from build123d import *

# Parameters (mm, degrees)
SKETCH1_R           = 9.525
BOSS_EXTRUDE1_DEPTH = 7.62
SKETCH2_R           = 3.175
CUT_EXTRUDE1_DEPTH  = 16.476293161
CUT_SWEEP5_PITCH    = 4.98602


with BuildPart() as part:
    # Sketch1 → Boss-Extrude1 (new body)
    with BuildSketch(Plane.XY):
        with Locations(Location((0, 0, 0), (0, 0, 180))):
            Circle(SKETCH1_R)
    extrude(amount=BOSS_EXTRUDE1_DEPTH)

    # Sketch2 → Cut-Extrude1 (cut, through all)
    with BuildSketch(Plane.XY.offset(7.62)):
        Circle(SKETCH2_R)
    extrude(amount=-CUT_EXTRUDE1_DEPTH, mode=Mode.SUBTRACT)

    # Cut-Sweep5: arcs per turn and ends read off the stored shape
    # Cut-Sweep5: the profile of Sketch6 screwed along a left-hand helix through 2.5 turns, 12 arcs to a turn; built about Z, then put on its axis
    cut_sweep5_z = Axis((0, 0, 0), (0, 0, 1))
    cut_sweep5_corners = [(10.033, 2e-08, -1.522198128), (10.033, 2e-08, 1.525801872), (8.509, 1.7e-08, 0.255801872), (8.509, 1.7e-08, -0.252198128)]
    with BuildLine(mode=Mode.PRIVATE) as cut_sweep5_profile:
        Line(cut_sweep5_corners[0], cut_sweep5_corners[1])
        Line(cut_sweep5_corners[1], cut_sweep5_corners[2])
        Line(cut_sweep5_corners[2], cut_sweep5_corners[3])
        Line(cut_sweep5_corners[3], cut_sweep5_corners[0])
    cut_sweep5_cap = Face(cut_sweep5_profile.wire())
    cut_sweep5_turn_angles = [0, -15, -30, -45, -60, -75, -90, -105, -120, -135, -150, -165, -180, -195, -210, -225, -240, -255, -270, -285, -300, -315, -330, -345, -360]
    cut_sweep5_turn_weights = [1, 0.9659258262890683, 1, 0.9659258262890683, 1, 0.9659258262890683, 1, 0.9659258262890683, 1, 0.9659258262890683, 1, 0.9659258262890683, 1, 0.9659258262890683, 1, 0.9659258262890683, 1, 0.9659258262890683, 1, 0.9659258262890683, 1, 0.9659258262890683, 1, 0.9659258262890683, 1]
    cut_sweep5_turn_rails = [Edge.make_bspline([Vector(p[0], p[1], 0).rotate(cut_sweep5_z, cut_sweep5_turn_angles[k]) / cut_sweep5_turn_weights[k] + Vector(0, 0, p[2] + -CUT_SWEEP5_PITCH * cut_sweep5_turn_angles[k] / 360) for k in range(25)], [0, 0, 0, 1, 1, 2, 2, 3, 3, 4, 4, 5, 5, 6, 6, 7, 7, 8, 8, 9, 9, 10, 10, 11, 11, 12, 12, 12], 2, cut_sweep5_turn_weights) for p in cut_sweep5_corners]
    cut_sweep5_turn_sides = [Face.make_surface_from_curves(cut_sweep5_turn_rails[p[0]], cut_sweep5_turn_rails[p[1]]) for p in [(0, 1), (1, 2), (2, 3), (3, 0)]]
    cut_sweep5_last_angles = [-720, -735, -750, -765, -780, -795, -810, -825, -840, -855, -870, -885, -900]
    cut_sweep5_last_weights = [1, 0.9659258262890683, 1, 0.9659258262890683, 1, 0.9659258262890683, 1, 0.9659258262890683, 1, 0.9659258262890683, 1, 0.9659258262890683, 1]
    cut_sweep5_last_rails = [Edge.make_bspline([Vector(p[0], p[1], 0).rotate(cut_sweep5_z, cut_sweep5_last_angles[k]) / cut_sweep5_last_weights[k] + Vector(0, 0, p[2] + -CUT_SWEEP5_PITCH * cut_sweep5_last_angles[k] / 360) for k in range(13)], [0, 0, 0, 1, 1, 2, 2, 3, 3, 4, 4, 5, 5, 6, 6, 6], 2, cut_sweep5_last_weights) for p in cut_sweep5_corners]
    cut_sweep5_last_sides = [Face.make_surface_from_curves(cut_sweep5_last_rails[p[0]], cut_sweep5_last_rails[p[1]]) for p in [(0, 1), (1, 2), (2, 3), (3, 0)]]
    cut_sweep5 = Plane(origin=(0, 0, 0), x_dir=(1, 0, 0), z_dir=(0, 0, 1)) * Solid(Shell([*[p.moved(Location((0, 0, CUT_SWEEP5_PITCH * i))) for i in range(2) for p in cut_sweep5_turn_sides], *cut_sweep5_last_sides, cut_sweep5_cap, cut_sweep5_cap.rotate(cut_sweep5_z, -900).moved(Location((0, 0, -CUT_SWEEP5_PITCH * -900 / 360)))]))
    add(cut_sweep5, mode=Mode.SUBTRACT)


solid = part.part
Source: CAD feature listing. Evaluate the final solid. Frame: model axes, mm. Coordinates: 2 decimals unless noted, no trailing zeros. Use a Markdown table: item, result.
1) Mould query, pull axis X, two halves, no side actions, for faces 1 (the flat face through (9.1, 0, 0.4)), 2 (the cylindrical face through (-0.69, -3.1, 3.86)). Classes: pulls with the +X half, pulls with the -X half, needs draft (parallel to the pull), parting line crosses it, or undercut.
Conclusion:
| item | result |
|---|---|
| face 1 | needs draft |
| face 2 | undercut |
2) First-contact query: pin 1 Ø4 at (x, z) = (-3, 6.5) entering from -Y; pin 2 Ø3 at (y, z) = (-7, 4) entering from -X; pin 3 Ø2 at (x, z) = (7.5, 1.5) entering from -Y. Flat tips, straight axial feed; report the tip coordinate or a pass-through.
Conclusion:
| item | result |
|---|---|
| pin 1 | stops at y = -9.44 |
| pin 2 | stops at x = -7.78 |
| pin 3 | stops at y = -6.93 |
3) Ray query, L1, parallel to Y at x = 0, z = 5.5 (3 decimals); L2, parallel to Y at x = 2.75, z = 2.5; L3, parallel to X at y = 8.75, z = 5.5. Return the intervals inside material, ascending.
Conclusion:
| item | result |
|---|---|
| L1 | y = -9.085 to -3.175, 3.175 to 9.525 |
| L2 | y = -9.12 to -1.59, 1.59 to 9.12 |
| L3 | x = -3.76 to 3.76 |
